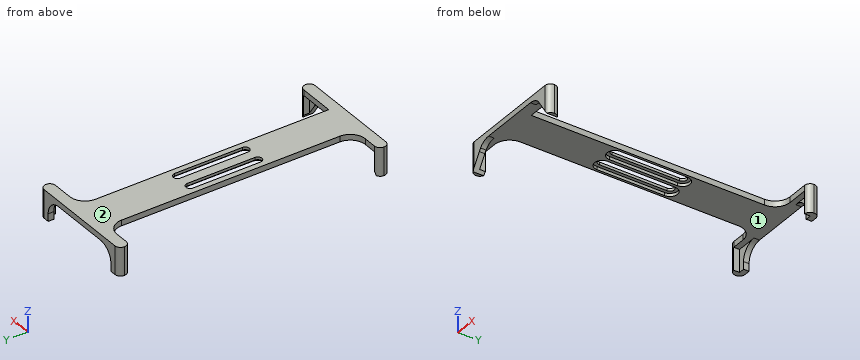
from build123d import *

# Parameters (mm, degrees)
BOSS_EXTRUDE1_DEPTH = 7.5
BOSS_EXTRUDE2_DEPTH = 30
FILLET1_R           = 20
FILLET2_R           = 20
FILLET4_R           = 7.5
CUT_EXTRUDE1_DEPTH  = 363.336169875
CUT_EXTRUDE2_DEPTH  = 4
CHAMFER1_START      = -352.5
CHAMFER1_DEPTH      = 15.5
CHAMFER1_2_DEPTH    = 7.3


with BuildPart() as part:
    # Sketch1 → Boss-Extrude1 (new body)
    with BuildSketch(Plane.XY):
        Polygon((-75, -337.5), (-30, -337.5), (-30, -7.5), (-75, -7.5), (-75, 7.5), (75, 7.5), (75, -7.5), (20, -7.5), (20, -337.5), (75, -337.5), (75, -352.5), (-75, -352.5), align=None)
    extrude(amount=BOSS_EXTRUDE1_DEPTH)

    # Sketch2 → Boss-Extrude2 (add)
    with BuildSketch(Plane(origin=(0, 0, 0), x_dir=(-1, 0, 0), z_dir=(0, 0, -1))):
        Polygon((67.7, -337.5), (67.7, -345.2), (60, -345.2), (60, -352.5), (75, -352.5), (75, -337.5), align=None)
        Polygon((-67.7, -337.5), (-67.7, -345.2), (-60, -345.2), (-60, -352.5), (-75, -352.5), (-75, -337.5), align=None)
        Polygon((-67.7, -7.5), (-75, -7.5), (-75, 7.5), (-60, 7.5), (-60, 0), (-67.7, 0), align=None)
        Polygon((67.7, -7.5), (75, -7.5), (75, 7.5), (60, 7.5), (60, 0.2), (67.7, 0.2), align=None)
    extrude(amount=BOSS_EXTRUDE2_DEPTH)

    # Fillet1
    fillet1_edges = [part.edges().sort_by_distance(p)[0] for p in [
        (-60, -348.85, 0),
        (60, -348.85, 0),
        (60, 3.75, 0),
        (-60, 3.85, 0),
    ]]
    fillet(fillet1_edges, radius=FILLET1_R)

    # Fillet2
    fillet2_edges = [part.edges().sort_by_distance(p)[0] for p in [
        (20, -7.5, 3.75),
        (-30, -337.5, 3.75),
        (-30, -7.5, 3.75),
    ]]
    fillet(fillet2_edges, radius=FILLET2_R)

    # Fillet4
    fillet4_edges = [part.edges().sort_by_distance(p)[0] for p in [
        (-75, -352.5, -11.25),
        (-75, -337.5, -11.25),
        (-75, -7.5, -11.25),
        (-75, 7.5, -11.25),
        (75, 7.5, -11.25),
        (75, -7.5, -11.25),
        (75, -337.5, -11.25),
        (75, -352.5, -11.25),
    ]]
    fillet(fillet4_edges, radius=FILLET4_R - 0.0001)  # a hair under: the kernel refuses the full size

    # Sketch3 → Cut-Extrude1 (cut, through all)
    with BuildSketch(Plane.XY.offset(7.5)):
        with BuildLine():
            Line((-22.5, -217.5), (-22.5, -127.5))
            ThreePointArc((-22.5, -127.5), (-17, -122), (-11.5, -127.5))
            Line((-11.5, -127.5), (-11.5, -217.5))
            ThreePointArc((-11.5, -217.5), (-17, -223), (-22.5, -217.5))
        make_face()
        with BuildLine():
            Line((1.5, -217.5), (1.5, -127.5))
            ThreePointArc((1.5, -127.5), (7, -122), (12.5, -127.5))
            Line((12.5, -127.5), (12.5, -217.5))
            ThreePointArc((12.5, -217.5), (7, -223), (1.5, -217.5))
        make_face()
    extrude(amount=-CUT_EXTRUDE1_DEPTH, mode=Mode.SUBTRACT)

    # Sketch4 → Cut-Extrude2 (cut)
    with BuildSketch(Plane(origin=(0, 0, 0), x_dir=(-1, 0, 0), z_dir=(0, 0, -1))):
        with BuildLine():
            Line((27, -127.5), (27, -217.5))
            ThreePointArc((27, -217.5), (17, -227.5), (7, -217.5))
            Line((7, -217.5), (7, -127.5))
            ThreePointArc((7, -127.5), (17, -117.5), (27, -127.5))
        make_face()
        with BuildLine():
            Line((3, -127.5), (3, -217.5))
            ThreePointArc((3, -217.5), (-7, -227.5), (-17, -217.5))
            Line((-17, -217.5), (-17, -127.5))
            ThreePointArc((-17, -127.5), (-7, -117.5), (3, -127.5))
        make_face()
    extrude(amount=-CUT_EXTRUDE2_DEPTH, mode=Mode.SUBTRACT)

    # Chamfer1: read off the stored shape, not the designer's step
    # Chamfer1 outline → Chamfer1 (cut)
    with BuildSketch(Plane(origin=(0, 0, 0), x_dir=(1, 0, 0), z_dir=(0, 1, 0)).offset(CHAMFER1_START)):
        with BuildLine():
            Line((70.453642879, 30), (60, 30))
            Line((60, 30), (60, 20))
            ThreePointArc((60, 20), (59.425347085, 15.240179557), (57.734410936, 10.753883584))
            Line((57.734410936, 10.753883584), (70.453642879, 30))
        make_face()
        with BuildLine():
            ThreePointArc((-57.734410936, 10.753883584), (-59.425347085, 15.240179557), (-60, 20))
            Line((-60, 20), (-60, 30))
            Line((-60, 30), (-70.453642879, 30))
            Line((-70.453642879, 30), (-57.734410936, 10.753883584))
        make_face()
    extrude(amount=CHAMFER1_DEPTH, mode=Mode.SUBTRACT)

    # Chamfer1 2 outline → Chamfer1 2 (add)
    with BuildSketch(Plane(origin=(0, 0, 0), x_dir=(1, 0, 0), z_dir=(0, 1, 0)).offset(CHAMFER1_START)):
        with BuildLine():
            ThreePointArc((55.458381501, 7.309907748), (56.685490998, 8.973015363), (57.734410936, 10.753883584))
            Line((57.734410936, 10.753883584), (55.458381501, 7.309907748))
        make_face()
        with BuildLine():
            ThreePointArc((-57.734410936, 10.753883584), (-56.685490998, 8.973015363), (-55.458381501, 7.309907748))
            Line((-55.458381501, 7.309907748), (-57.734410936, 10.753883584))
        make_face()
    extrude(amount=CHAMFER1_2_DEPTH)


solid = part.part
Here's how the part is built. I have some questions about the finished solid (model axes, mm). Face numbers are marked on the shaded views. Round coordinates to 2 decimals unless told otherwise and drop trailing zeros. Write each loop counter-clockwise with the first axis right and the second up, starting at its lowest first coordinate (ties: lowest second). Pieces come first, ordered by that corner, then holes.
1. If we mould it in two halves opening along X, with no side actions, what happens to the marked faces 1 and 2? For each: released by +X, released by -X, zero draft, split by the parting line, or undercut.
2. I need wall thicknesses on L1, parallel to Y at x = 65, z = -6.5; L2, parallel to Z at x = -5.5, y = -153.5; L3, parallel to Y at x = -63.5, z = -7. Which ranges of each line are inside material? Lowest first, please.
3. Will these pins go through, and if not, where does the flat tip stop? pin 1 Ø8 at (y, z) = (-174.5, 2) entering from +X; pin 2 Ø6 at (x, y) = (-15.5, -157.5) entering from -Z; pin 3 Ø6 at (y, z) = (-340.5, -14) entering from -X; pin 4 Ø2 at (y, z) = (5, -23) entering from +X.
4. Suppose I cut it at C-C (y = -40.5). List the corners of the cut face in (x, z) for me, and give its area (3 significant figures).
5. Suppose I cut it at D-D (x = 27). List the corners of the cut face in (y, z) for me.
6. Suppose I cut it at A-A (x = -17). List the corners of the cut face in (y, z) for me, and give its area (3 significant figures).
7. Suppose I cut it at B-B (z = -16). State how many separate pieces and enclosed holes the cut face has, and give its area (3 significant figures).
Answer sheet:
1. face 1: undercut
1. face 2: zero draft
2. L1: y = -352.5 to -345.2, 0 to 7.5
2. L2: z = 0 to 7.5
2. L3: y = -352.5 to -345.2, 0.2 to 7.5
3. pin 1: stops at x = 20
3. pin 2: passes through
3. pin 3: stops at x = -74.85
3. pin 4: stops at x = 73.84
4. outline: (-30, 0) - (20, 0) - (20, 7.5) - (-30, 7.5) - close
4. area: 375 mm2
5. outline: (-352.5, 0) - (-337.5, 0) - (-337.5, 7.5) - (-352.5, 7.5) - close; (-12.3, 0) - (7.5, 0) - (7.5, 7.5) - (-12.3, 7.5) - close
6. outline: (-352.5, 0) - (-227.5, 0) - (-227.5, 4) - (-223, 4) - (-223, 7.5) - (-352.5, 7.5) - close; (-122, 4) - (-117.5, 4) - (-117.5, 0) - (7.5, 0) - (7.5, 7.5) - (-122, 7.5) - close
6. area: 1,910 mm2
7. separate pieces: 4
7. enclosed holes: 0
7. area: 556 mm2
